Read the model definition and answer for the solid it produces. Units are mm, in the model's axes. A direction names the side the tool comes from. Give positions to 0.01 mm unless a question says otherwise; leave off trailing zeros. Order: outer loops, then holes, each group sorted by start corner. A loop starts at its lowest first (then second) coordinate and runs counter-clockwise, first axis right, second up. Notation, with made-up numbers: (60, 53) - (98, 53) arc R17 cw to (98, 79) - close; hole circle Ø5 at (-0.5, 32.25). An arc over 180 degrees is marked (long way). One line per item, written item: value. Start each with the question number.
```python
from build123d import *

# Parameters (mm, degrees)
F1_DEPTH = 46
F3_D     = 6
F5_R     = 6
F6_SIZE  = 2
F4_R     = 4.5
F7_DEPTH = 25


with BuildPart() as f1:
    # F0 (on Right) → F1 (new body)
    with BuildSketch(Plane.YZ):
        Polygon((56.5, 0), (0, 0), (0, -52), (6, -52), (6, -6), (56.5, -6), align=None)
    extrude(amount=F1_DEPTH)

    # F3 (through all)
    with Locations(Plane.XY):
        with Locations((13.5, 16.9), (32.5, 16.9), (32.5, 48.7), (13.5, 48.7)):
            Hole(F3_D / 2)

    # F5
    f5_edges = [f1.edges().sort_by_distance(p)[0] for p in [
        (23, 0, 0),
    ]]
    fillet(f5_edges, radius=F5_R)

    # F6
    f6_edges = [f1.edges().sort_by_distance(p)[0] for p in [
        (46, 56.5, -3),
        (0, 56.5, -3),
        (0, 3, -52),
        (46, 3, -52),
    ]]
    chamfer(f6_edges, length=F6_SIZE)

    # F4 (on face) → F7 (cut)
    with BuildSketch(Plane.XZ):
        with Locations((23, -19)):
            Circle(F4_R)
        with BuildLine():
            ThreePointArc((23, -37.5), (16.672627, -36.384313), (11.108429, -33.171822))
            ThreePointArc((11.108429, -33.171822), (4.768685, -33.726478), (5.323341, -40.066222))
            ThreePointArc((5.323341, -40.066222), (13.594446, -44.841547), (23, -46.5))
            ThreePointArc((23, -46.5), (27.5, -42), (23, -37.5))
        make_face()
    extrude(amount=-F7_DEPTH, mode=Mode.SUBTRACT)


solid = f1.part
```
1) The mould has two halves that part along X. Classify faces 1 (the flat face through (46, 15, -5)), 2 (the flat face through (1, 3, -51)), 3 (the flat face through (23, 31, -6)), 4 (the cylindrical face through (14.15, 13.97, -3.04)): +X half, -X half, draft (parallel to the pull), parting line (faces both ways), or undercut.
2) Each of these flat-tipped pins is pushed along its axis until it touches: pin 1 (23 mm diameter, centred on x = 14, y = 42.5, fed in from -Z); pin 2 (14 mm diameter, centred on x = 16, z = -29.5, fed in from +Y). Where does it stop, or does it pass through?
3) Section A-A on z = -19 is taken. Write down the section's boundary in (x, y), plus the area to 3 significant figures.
4) For faces 5 (the cylindrical face through (13.468, 2.958, -44.795)), 6 (the flat face through (23, 6, -29)), 7 (the flat face through (45, 55.5, -3)), determine the directions among +Z, -Z, +X, -X, +Y, -Y from which every point of the face is accessible in a straight line to the end or side of a thin tool.
5) Section C-C on x = 25 is taken. Write down the section's boundary in (y, z), plus the area to 3 significant figures.
6) Section B-B on y = 16.9 is taken. Write down the section's boundary in (x, z).
7) Section D-D on z = -4 is taken. Write down the section's boundary in (x, y), plus the area to 3 significant figures.
8) Find the intervals of material crossed by probe 1 along Y at (x, z) = (32.5, -4.5); probe 2 along X at (y, z) = (48, -2); probe 3 along Y at (x, z) = (32.5, -3.6), in increasing order. Write a range as from..to.
Solved:
1. face 1: +X half
1. face 2: -X half
1. face 3: draft
1. face 4: undercut
2. pin 1: stops at z = -6
2. pin 2: stops at y = 6
3. outline: (0, 0) - (18.5, 0) - (18.5, 6) - (0, 6) - close; (27.5, 0) - (46, 0) - (46, 6) - (27.5, 6) - close
3. area: 222 mm2
4. face 5: +Y, -Y
4. face 6: -Z, +X, -X, +Y
4. face 7: +Z, -Z, +X, +Y
5. outline: (0, -52) - (6, -52) - (6, -46.03) - (0, -46.03) - close; (0, -37.97) - (6, -37.97) - (6, -23.03) - (0, -23.03) - close; (0, -14.97) - (6, -14.97) - (6, -6) - (56.5, -6) - (56.5, 0) - (6, 0) arc R6 ccw to (0, -6) - close
5. area: 511 mm2
6. outline: (0, -6) - (10.5, -6) - (10.5, 0) - (0, 0) - close; (16.5, -6) - (29.5, -6) - (29.5, 0) - (16.5, 0) - close; (35.5, -6) - (46, -6) - (46, 0) - (35.5, 0) - close
7. outline: (0, 0.34) - (46, 0.34) - (46, 54.5) - (44, 56.5) - (2, 56.5) - (0, 54.5) - close; hole circle Ø6 at (13.5, 16.9); hole circle Ø6 at (13.5, 48.7); hole circle Ø6 at (32.5, 16.9); hole circle Ø6 at (32.5, 48.7)
7. area: 2,470 mm2
8. probe 1: y = 0.19..13.9, 19.9..45.7, 51.7..56.5
8. probe 2: x = 0..10.58, 16.42..29.58, 35.42..46
8. probe 3: y = 0.5..13.9, 19.9..45.7, 51.7..56.5
